```python
from build123d import *

# Parameters (mm, degrees)
F0_R     = 5
F1_DEPTH = 769.17
F2_R     = 4
F3_DEPTH = 2.5


with BuildPart() as f1:
    # F0 (on Right) → F1 (new body)
    with BuildSketch(Plane.YZ):
        Circle(F0_R)
    extrude(amount=F1_DEPTH)

    # F2 (on Front) → F3 (join, symmetric)
    with BuildSketch(Plane.XZ):
        with BuildLine():
            Line((0, -6), (0, 6))
            Line((0, 6), (-8.708497, 6))
            ThreePointArc((-8.708497, 6), (-22, 0), (-8.708497, -6))
            Line((-8.708497, -6), (0, -6))
        make_face()
        with Locations((-14, 0)):
            Circle(F2_R, mode=Mode.SUBTRACT)
        with BuildLine():
            Line((777.878497, 6), (769.17, 6))
            Line((769.17, 6), (769.17, -6))
            Line((769.17, -6), (777.878497, -6))
            ThreePointArc((777.878497, -6), (791.17, 0), (777.878497, 6))
        make_face()
        with Locations((783.17, 0)):
            Circle(F2_R, mode=Mode.SUBTRACT)
    extrude(amount=F3_DEPTH, both=True)


solid = f1.part
```
Input: part model. Units: mm. Frame: model coordinates. A direction names the side the tool comes from. Coordinates: 2 decimals unless noted, no trailing zeros. Write each loop counter-clockwise with the first axis right and the second up, starting at its lowest first coordinate (ties: lowest second). Pieces come first, ordered by that corner, then holes.
1) Section B-B on y = 0. Output: boundary loops of the cut face in (x, z).
2) Set-up query: faces 1 (the flat face through (778, -2.5, 0)), 2 (the flat face through (-9, 2.5, 0)), 3 (the flat face through (778, 2.5, 0)), 4 (the cylindrical face through (-22, 0, 0)). Return all of +Z, -Z, +X, -X, +Y, -Y with unobstructed straight access to the full face (end or side cutting, diameter ignored); none if empty.
3) Material intervals for line 1 along Z through (x, y) = (-14, -0.9); line 2 along Y through (x, z) = (159, 1); line 3 along Y through (x, z) = (56.5, 4.25), sorted ascending.
4) Mould query, pull axis X, two halves, no side actions, for faces 5 (the flat face through (-9, -2.5, 0)), 6 (the cylindrical face through (791.166, -0.035, -0.257)). Classes: pulls with the +X half, pulls with the -X half, needs draft (parallel to the pull), parting line crosses it, or undercut.
5) Section C-C on x = 671. Output: boundary loops of the cut face in (y, z).
6) Section A-A on z = 0. Output: boundary loops of the cut face in (x, y).
7) Pin query (flat end, axial travel): pin 1 Ø3 at (y, z) = (2.5, 2) entering from +X; pin 2 Ø8 at (x, z) = (130, -3) entering from -Y; pin 3 Ø1.5 at (x, y) = (772.5, -0.5) entering from -Z; pin 4 Ø2 at (y, z) = (-4, -1.5) entering from +X. Return the tip coordinate at first contact, or that it passes through.
Check result:
1. outline: (-8.71, -6) - (0, -6) - (0, -5) - (769.17, -5) - (769.17, -6) - (777.88, -6) arc R8 ccw (long way) to (777.88, 6) - (769.17, 6) - (769.17, 5) - (0, 5) - (0, 6) - (-8.71, 6) arc R8 ccw (long way) to start; hole circle Ø8 at (-14, 0); hole circle Ø8 at (783.17, 0)
2. face 1: +Z, -Z, +X, -Y
2. face 2: +Z, -Z, -X, +Y
2. face 3: +Z, -Z, +X, +Y
2. face 4: +Y, -Y
3. line 1: z = -8 to -4, 4 to 8
3. line 2: y = -4.9 to 4.9
3. line 3: y = -2.63 to 2.63
4. face 5: needs draft
4. face 6: undercut
5. outline: circle Ø10 at (0, 0)
6. outline: (-22, -2.5) - (-18, -2.5) - (-18, 2.5) - (-22, 2.5) - close; (-10, -2.5) - (0, -2.5) - (0, -5) - (769.17, -5) - (769.17, -2.5) - (779.17, -2.5) - (779.17, 2.5) - (769.17, 2.5) - (769.17, 5) - (0, 5) - (0, 2.5) - (-10, 2.5) - close; (787.17, -2.5) - (791.17, -2.5) - (791.17, 2.5) - (787.17, 2.5) - close
7. pin 1: stops at x = 791.15
7. pin 2: stops at y = -5
7. pin 3: stops at z = -6
7. pin 4: stops at x = 769.17
